Design review of the part built by this model. Coordinates are the model's own, in mm. A direction names the side the tool comes from. Coordinates: 2 decimals unless noted, no trailing zeros. Loops run counter-clockwise (first coordinate to the right, second up) from the corner with the lowest first, then second, coordinate; pieces in that order, holes last. Notation, with made-up numbers: (83.25, -21.5) -> (108.25, -21.5) arc R17 ccw to (108.25, 4.5) -> close; hole circle Ø1 at (-28, -29). An arc over 180 degrees is marked (long way). One line per item, written item: value. Start each with the question number.
1. Machinability: for faces 1 (the flat face through (-402.817, -8.653, 52.568)), 2 (the flat face through (-415.03, 3.45, 44.62)), 3 (the cylindrical face through (-410.98, -8.65, 44.75)), 4 (the flat face through (-400, 0, 51)), which of the approach directions +Z, -Z, +X, -X, +Y, -Y give a long, thin tool a straight path to every point of the face, cutting with its end or side? Answer none if there is none.
2. Insertion check: pin 1 (4 mm diameter, centred on y = -6, z = 51, fed in from -X); pin 2 (2 mm diameter, centred on x = -401.5, z = 45, fed in from +Y); pin 3 (1.5 mm diameter, centred on y = 3, z = 53.5, fed in from +X); pin 4 (12 mm diameter, centred on y = -2, z = 65.5, fed in from +X). Each pin has a flat end and moves straight along its axis. Give the tip position at first contact, or say it passes through.
3. Add section B-B on z = 67. Write out the cut boundary in (x, y) (3 decimals), plus the area to 3 significant figures.
4. For probe 1 along Y at (x, z) = (-401.25, 52) (3 decimals); probe 2 along Y at (x, z) = (-399, 68) (3 decimals); probe 3 along X at (y, z) = (6.25, 63), list the stretches that pass through material, from the lowest coordinate up.
5. Add section A-A on y = -9. Write out the cut boundary in (x, z).
```python
from build123d import *

# Parameters (mm, degrees)
BOSS_EXTRUDE1_DEPTH = 7
BOSS_EXTRUDE3_START = 3.175
BOSS_EXTRUDE3_DEPTH = 3.175
BOSS_EXTRUDE4_DEPTH = 12.7
FILLET2_R           = 1.5875


with BuildPart() as part:
    # Sketch1 → Boss-Extrude1 (new body)
    # profile 1 of 2: a face of its own
    with BuildSketch(Plane(origin=(0, 0, 0), x_dir=(1, 0, 0), z_dir=(0, 1, 0))):
        with BuildLine():
            Line((-397.046660629, -66.449724392), (-396.047807587, -65.58143469))
            ThreePointArc((-396.047807587, -65.58143469), (-394.269590942, -62.014883864), (-395.534134167, -58.235562542))
            Line((-395.534134167, -58.235562542), (-407.251348425, -44.756449439))
            ThreePointArc((-407.251348425, -44.756449439), (-410.81789925, -42.978232793), (-414.597220573, -44.242776019))
            Line((-414.597220573, -44.242776019), (-415.480745161, -45.010812225))
            ThreePointArc((-415.480745161, -45.010812225), (-417.25736044, -48.555145476), (-416.023502117, -52.322937096))
            Line((-416.023502117, -52.322937096), (-404.421616313, -65.902303694))
            ThreePointArc((-404.421616313, -65.902303694), (-400.848199526, -67.712666251), (-397.046660629, -66.449724392))
        make_face()
        with BuildLine():
            ThreePointArc((-396.131127084, -65.485586573), (-394.396281576, -62.006024792), (-395.629982284, -58.318882038))
            Line((-395.629982284, -58.318882038), (-407.347196542, -44.839768935))
            ThreePointArc((-407.347196542, -44.839768935), (-410.826758322, -43.104923427), (-414.513901076, -44.338624135))
            Line((-414.513901076, -44.338624135), (-415.397425664, -45.106660342))
            ThreePointArc((-415.397425664, -45.106660342), (-417.130708863, -48.564546441), (-415.926944646, -52.240440703))
            Line((-415.926944646, -52.240440703), (-404.325058842, -65.819807301))
            ThreePointArc((-404.325058842, -65.819807301), (-400.838798562, -67.586014674), (-397.129980126, -66.353876275))
            Line((-397.129980126, -66.353876275), (-396.131127084, -65.485586573))
        make_face(mode=Mode.SUBTRACT)
    # profile 2 of 2: a face of its own
    with BuildSketch(Plane(origin=(0, 0, 0), x_dir=(1, 0, 0), z_dir=(0, 1, 0))):
        with BuildLine():
            Line((-397.129980126, -66.353876275), (-396.131127084, -65.485586573))
            ThreePointArc((-396.131127084, -65.485586573), (-394.396281576, -62.006024792), (-395.629982284, -58.318882038))
            Line((-395.629982284, -58.318882038), (-407.347196542, -44.839768935))
            ThreePointArc((-407.347196542, -44.839768935), (-410.826758322, -43.104923427), (-414.513901076, -44.338624135))
            Line((-414.513901076, -44.338624135), (-415.397425664, -45.106660342))
            ThreePointArc((-415.397425664, -45.106660342), (-417.130708863, -48.564546441), (-415.926944646, -52.240440703))
            Line((-415.926944646, -52.240440703), (-404.325058842, -65.819807301))
            ThreePointArc((-404.325058842, -65.819807301), (-400.838798562, -67.586014674), (-397.129980126, -66.353876275))
        make_face()
    extrude(amount=BOSS_EXTRUDE1_DEPTH)

    # Sketch3 → Boss-Extrude3 (add)
    # profile 1 of 2: a face of its own
    with BuildSketch(Plane.XZ.offset(BOSS_EXTRUDE3_START)):
        with BuildLine():
            Line((-393.881500674, 68.073485724), (-394.880353715, 68.941775426))
            ThreePointArc((-394.880353715, 68.941775426), (-401.092624596, 71.005607244), (-406.932110565, 68.047209895))
            Line((-406.932110565, 68.047209895), (-418.533996369, 54.467843297))
            ThreePointArc((-418.533996369, 54.467843297), (-420.550301433, 48.310720407), (-417.647052074, 42.518761191))
            Line((-417.647052074, 42.518761191), (-416.763527487, 41.750724985))
            ThreePointArc((-416.763527487, 41.750724985), (-410.587563374, 39.684276299), (-404.759297391, 42.590142525))
            Line((-404.759297391, 42.590142525), (-393.042083133, 56.069255628))
            ThreePointArc((-393.042083133, 56.069255628), (-390.975634448, 62.245219741), (-393.881500674, 68.073485724))
        make_face()
        with BuildLine():
            Line((-396.047807587, 65.58143469), (-397.046660629, 66.449724392))
            ThreePointArc((-397.046660629, 66.449724392), (-400.848199526, 67.712666251), (-404.421616313, 65.902303694))
            Line((-404.421616313, 65.902303694), (-416.023502117, 52.322937096))
            ThreePointArc((-416.023502117, 52.322937096), (-417.25736044, 48.555145476), (-415.480745161, 45.010812225))
            Line((-415.480745161, 45.010812225), (-414.597220573, 44.242776019))
            ThreePointArc((-414.597220573, 44.242776019), (-410.81789925, 42.978232793), (-407.251348425, 44.756449439))
            Line((-407.251348425, 44.756449439), (-395.534134167, 58.235562542))
            ThreePointArc((-395.534134167, 58.235562542), (-394.269590942, 62.014883864), (-396.047807587, 65.58143469))
        make_face(mode=Mode.SUBTRACT)
    # profile 2 of 2: a face of its own
    with BuildSketch(Plane.XZ.offset(BOSS_EXTRUDE3_START)):
        with BuildLine():
            ThreePointArc((-395.534134167, 58.235562542), (-394.269590942, 62.014883864), (-396.047807587, 65.58143469))
            Line((-396.047807587, 65.58143469), (-397.046660629, 66.449724392))
            ThreePointArc((-397.046660629, 66.449724392), (-400.848199526, 67.712666251), (-404.421616313, 65.902303694))
            Line((-404.421616313, 65.902303694), (-416.023502117, 52.322937096))
            ThreePointArc((-416.023502117, 52.322937096), (-417.25736044, 48.555145476), (-415.480745161, 45.010812225))
            Line((-415.480745161, 45.010812225), (-414.597220573, 44.242776019))
            ThreePointArc((-414.597220573, 44.242776019), (-410.81789925, 42.978232793), (-407.251348425, 44.756449439))
            Line((-407.251348425, 44.756449439), (-395.534134167, 58.235562542))
        make_face()
    extrude(amount=-BOSS_EXTRUDE3_DEPTH)

    # Sketch4 → Boss-Extrude4 (add)
    with BuildSketch(Plane.XZ.offset(3.175)):
        with BuildLine():
            Line((-397.214280541, 64.239561056), (-398.213133583, 65.107850758))
            ThreePointArc((-398.213133583, 65.107850758), (-400.716586027, 65.939544178), (-403.069811716, 64.747354201))
            Line((-403.069811716, 64.747354201), (-414.67169752, 51.167987603))
            ThreePointArc((-414.67169752, 51.167987603), (-415.484238367, 48.686758975), (-414.314272207, 46.352685859))
            Line((-414.314272207, 46.352685859), (-413.430747619, 45.584649652))
            ThreePointArc((-413.430747619, 45.584649652), (-410.941926261, 44.751901674), (-408.593222058, 45.922922392))
            Line((-408.593222058, 45.922922392), (-396.876007801, 59.402035495))
            ThreePointArc((-396.876007801, 59.402035495), (-396.043259823, 61.890856854), (-397.214280541, 64.239561056))
        make_face()
    extrude(amount=BOSS_EXTRUDE4_DEPTH)

    # Fillet2
    fillet2_edges = [part.edges().sort_by_distance(p)[0] for p in [
        (-397.713707062, -15.875, 64.673705907),
        (-400.716586027, -15.875, 65.939544178),
        (-408.870754618, -15.875, 57.957670902),
        (-415.484238367, -15.875, 48.686758975),
        (-413.872509913, -15.875, 45.968667755),
        (-410.941926261, -15.875, 44.751901674),
        (-402.73461493, -15.875, 52.662478944),
        (-396.043259823, -15.875, 61.890856854),
    ]]
    fillet(fillet2_edges, radius=FILLET2_R)


solid = part.part
```
Worked answers:
1. face 1: -Z, +X, -Y
1. face 2: -Z, -X, +Y
1. face 3: -Z, -Y
1. face 4: +Y
2. pin 1: stops at x = -415.49
2. pin 2: stops at y = 0
2. pin 3: stops at x = -399
2. pin 4: stops at x = -390.95
3. outline: (-407.827, -3.175) -> (-392.846, -3.175) -> (-392.846, 0) -> (-397.809, 0) -> (-397.809, 7) -> (-403.116, 7) -> (-403.116, 0) -> (-407.827, 0) -> close
3. area: 84.7 mm²
4. probe 1: y = -3.175 to 7
4. probe 2: y = -3.175 to 0
4. probe 3: x = -406.9 to -394.43
5. outline: (-414.67, 51.17) arc R3.43 ccw to (-414.31, 46.35) -> (-413.43, 45.58) arc R3.43 ccw to (-408.59, 45.92) -> (-396.88, 59.4) arc R3.43 ccw to (-397.21, 64.24) -> (-398.21, 65.11) arc R3.43 ccw to (-403.07, 64.75) -> close
